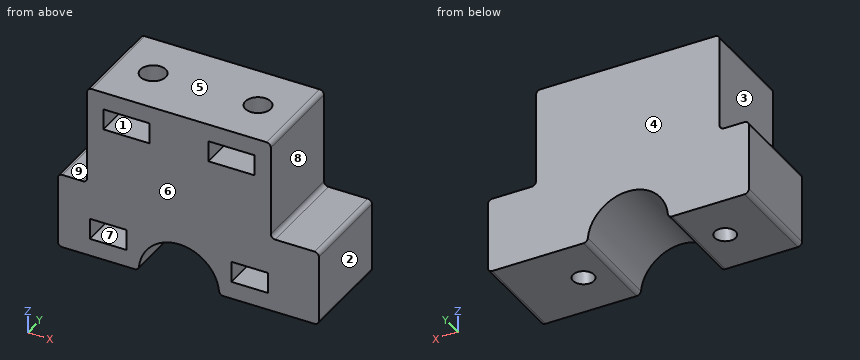
from build123d import *

# Parameters (mm, degrees)
BOSS_EXTRUDE1_DEPTH = 11
SKETCH2_R           = 1.45
CUT_EXTRUDE1_DEPTH  = 8
SKETCH3_R           = 1.2
CUT_EXTRUDE2_DEPTH  = 10
CUT_EXTRUDE3_START  = -2
SKETCH5_R           = 1.2
CUT_EXTRUDE3_DEPTH  = 2.4
CUT_EXTRUDE4_START  = -2
CUT_EXTRUDE4_DEPTH  = 2.4
SKETCH1_4_W         = 5.5
SKETCH1_4_H         = 8.65
SKETCH1_4_W_2       = 3.35
BOSS_EXTRUDE2_DEPTH = 11
FILLET2_R           = 0.5


with BuildPart() as part:
    # Sketch1 → Boss-Extrude1 (new body)
    with BuildSketch(Plane(origin=(0, 0, 0), x_dir=(1, 0, 0), z_dir=(0, 1, 0))):
        with BuildLine():
            ThreePointArc((-4.6, 10), (0, 5.4), (4.6, 10))
            Line((4.6, 10), (10.5, 10))
            Line((10.5, 10), (10.5, -10))
            Line((10.5, -10), (-10.5, -10))
            Line((-10.5, -10), (-10.5, 10))
            Line((-10.5, 10), (-4.6, 10))
        make_face()
    extrude(amount=BOSS_EXTRUDE1_DEPTH)

    # Sketch2 → Cut-Extrude1 (cut)
    with BuildSketch(Plane.XY.offset(10)):
        with Locations((-6, 5.5)):
            Circle(SKETCH2_R)
        with Locations((6, 5.5)):
            Circle(SKETCH2_R)
    extrude(amount=-CUT_EXTRUDE1_DEPTH, mode=Mode.SUBTRACT)

    # Sketch3 → Cut-Extrude2 (cut)
    with BuildSketch(Plane(origin=(0, 0, -10), x_dir=(-1, 0, 0), z_dir=(0, 0, -1))):
        with Locations((-8.1, 5.5)):
            Circle(SKETCH3_R)
        with Locations((8.1, 5.5)):
            Circle(SKETCH3_R)
    extrude(amount=-CUT_EXTRUDE2_DEPTH, mode=Mode.SUBTRACT)

    # Sketch5 → Cut-Extrude3 (cut)
    # profile 1 of 2: a face of its own
    with BuildSketch(Plane(origin=(0, 0, -10), x_dir=(-1, 0, 0), z_dir=(0, 0, -1)).offset(CUT_EXTRUDE3_START)):
        Polygon((-6, 0), (-6, 4.287564435), (-6, 6.712435565), (-8.1, 7.924871131), (-10.2, 6.712435565), (-10.2, 4.287564435), (-10.2, 0), align=None)
        with Locations((-8.1, 5.5)):
            Circle(SKETCH5_R, mode=Mode.SUBTRACT)
    # profile 2 of 2: a face of its own
    with BuildSketch(Plane(origin=(0, 0, -10), x_dir=(-1, 0, 0), z_dir=(0, 0, -1)).offset(CUT_EXTRUDE3_START)):
        Polygon((6, 0), (10.2, 0), (10.2, 4.287564435), (10.2, 6.712435565), (8.1, 7.924871131), (6, 6.712435565), (6, 4.287564435), align=None)
    extrude(amount=-CUT_EXTRUDE3_DEPTH, mode=Mode.SUBTRACT)

    # Sketch6 → Cut-Extrude4 (cut)
    with BuildSketch(Plane.XY.offset(10).offset(CUT_EXTRUDE4_START)):
        Polygon((-6, 8.559956427), (-8.65, 7.029978213), (-8.65, 3.970021787), (-8.65, 0), (-3.35, 0), (-3.35, 3.970021787), (-3.35, 7.029978213), align=None)
        Polygon((6, 8.559956427), (3.35, 7.029978213), (3.35, 3.970021787), (3.35, 0), (8.65, 0), (8.65, 3.970021787), (8.65, 7.029978213), align=None)
    extrude(amount=-CUT_EXTRUDE4_DEPTH, mode=Mode.SUBTRACT)

    # Sketch1<4> → Boss-Extrude2 (add, through all)
    with BuildSketch(Plane(origin=(0, 0, 0), x_dir=(1, 0, 0), z_dir=(0, 1, 0))):
        with Locations((13.25, 5.675)):
            Rectangle(SKETCH1_4_W, SKETCH1_4_H)
        with Locations((-12.175, 5.675)):
            Rectangle(SKETCH1_4_W_2, SKETCH1_4_H)
    extrude(amount=BOSS_EXTRUDE2_DEPTH)

    # Fillet2
    fillet2_edges = [part.edges().sort_by_distance(p)[0] for p in [
        (10.5, 5.5, -1.35),
        (16, 5.5, -1.35),
        (16, 5.5, -10),
        (4.6, 5.5, -10),
        (10.5, 5.5, 10),
        (-10.5, 5.5, 10),
        (-4.6, 5.5, -10),
        (-13.85, 5.5, -10),
        (-13.85, 5.5, -1.35),
        (-10.5, 5.5, -1.35),
    ]]
    fillet(fillet2_edges, radius=FILLET2_R)


solid = part.part
Source: CAD feature listing. Evaluate the final solid. Frame: model axes, mm. Face numbers are marked on the shaded views. A direction names the side the tool comes from. Round coordinates to 2 decimals unless told otherwise and drop trailing zeros. Loops run counter-clockwise (first coordinate to the right, second up) from the corner with the lowest first, then second, coordinate; pieces in that order, holes last.
Q1. Section A-A, the plane z = -2.75. Return loops of the section in (x, y).
Q2. Section D-D, the plane x = 12.5. Return loops of the section in (y, z).
Q3. Mould query, pull axis X, two halves, no side actions, for the marked faces 1, 2, 3 and 4. Classes: pulls with the +X half, pulls with the -X half, needs draft (parallel to the pull), parting line crosses it, or undercut.
Q4. Section C-C, the plane y = 3.25. State how many separate pieces and enclosed holes the cut face has, plus the area to 3 significant figures.
Q5. Access query for the marked faces 5, 6, 7, 8 and 9. Directions: +Z, -Z, +X, -X, +Y, -Y. A direction counts if a zero-diameter tool reaches every point of the face in a straight line with its end or side. Return the directions, or none.
Q6. Section B-B, the plane z = -6.25. Return loops of the section in (x, y), plus the area to 3 significant figures.
Q7. First-contact query: P1, Ø1.9, axis at y = 2, z = 6.5, coming from the +X side; P2, Ø0.7, axis at y = 3.5, z = 6.5, coming from the -X side; P3, Ø1, axis at y = 8, z = -1, coming from the -X side. Flat tips, straight axial feed; report the tip coordinate or a pass-through.
Q8. Ray query, line 1 (X direction, y = 6.25, z = 6); line 2 (Z direction, x = 7.5, y = 4); line 3 (X direction, y = 4.25, z = 4.25). Return the intervals inside material, ascending.
Solutions:
1. outline: (-13.85, 0) - (16, 0) - (16, 11) - (-13.85, 11) - close; hole circle Ø2.4 at (-8.1, 5.5); hole circle Ø2.4 at (8.1, 5.5)
2. outline: (0, -10) - (11, -10) - (11, -1.35) - (0, -1.35) - close
3. face 1: undercut
3. face 2: pulls with the +X half
3. face 3: pulls with the -X half
3. face 4: needs draft
4. separate pieces: 1
4. enclosed holes: 4
4. area: 417 mm2
5. face 5: +Z, +X, -X, +Y, -Y
5. face 6: +Z, -Z, +X, -X, -Y
5. face 7: -Y
5. face 8: +Z, +X, +Y, -Y
5. face 9: +Z, -X, +Y, -Y
6. outline: (-13.85, 0) - (-10.2, 0) - (-10.2, 6.71) - (-8.1, 7.92) - (-6, 6.71) - (-6, 0) - (-2.66, 0) - (-2.66, 11) - (-13.85, 11) - close; (2.66, 0) - (6, 0) - (6, 6.71) - (8.1, 7.92) - (10.2, 6.71) - (10.2, 0) - (16, 0) - (16, 11) - (2.66, 11) - close
6. area: 208 mm2
7. P1: stops at x = 10.5
7. P2: stops at x = -10.5
7. P3: stops at x = -13.71
8. line 1: x = -10.5 to -8.65, -3.35 to 3.35, 8.65 to 10.5
8. line 2: z = -10 to -8, -5.6 to 5.6, 8 to 10
8. line 3: x = -10.5 to -6.73, -5.27 to 5.27, 6.73 to 10.5
